```python
from build123d import *

# Parameters (mm, degrees)
BOSS_EXTRUDE1_DEPTH   = 3.81
LPATTERN1_COUNT       = 2
LPATTERN1_PITCH       = 60.96
BODY_MOVE_COPY1_ANGLE = 180
LPATTERN2_COUNT       = 3
LPATTERN2_PITCH       = 146.05
BODY_MOVE_COPY2_ANGLE = 120
BODY_MOVE_COPY3_ANGLE = 120
BOSS_EXTRUDE2_START   = -63.5
SKETCH2_R             = 9.5
BOSS_EXTRUDE2_DEPTH   = 480.06


with BuildPart() as part:
    # Sketch1 → Boss-Extrude1 (new, symmetric)
    with BuildSketch(Plane(origin=(0, 0, 0), x_dir=(1, 0, 0), z_dir=(0, 1, 0))):
        with BuildLine():
            Line((-5.499261314, 15.875), (-10.998522628, 6.35))
            ThreePointArc((-10.998522628, 6.35), (0, -12.7), (10.998522628, 6.35))
            Line((10.998522628, 6.35), (5.499261314, 15.875))
            ThreePointArc((5.499261314, 15.875), (0, 19.05), (-5.499261314, 15.875))
        make_face()
    extrude(amount=BOSS_EXTRUDE1_DEPTH, both=True)


with BuildPart() as lpattern1_1:
    # LPattern1: pattern copy
    add(part.part.moved(Location(Vector(0, 1, 0) * (1 * LPATTERN1_PITCH))))


with BuildPart() as lpattern1_1_1:
    # Body-Move/Copy1: moved
    add(lpattern1_1.part.rotate(Axis((0, 0, 0), (0, 1, 0)), BODY_MOVE_COPY1_ANGLE))


with BuildPart() as lpattern2_1:
    # LPattern2: pattern copy
    add(part.part.moved(Location(Vector(0, 1, 0) * (1 * LPATTERN2_PITCH))))


with BuildPart() as lpattern2_2:
    # LPattern2: pattern copy
    add(part.part.moved(Location(Vector(0, 1, 0) * (2 * LPATTERN2_PITCH))))


with BuildPart() as lpattern2_3:
    # LPattern2: pattern copy
    add(lpattern1_1_1.part.moved(Location(Vector(0, 1, 0) * (1 * LPATTERN2_PITCH))))


with BuildPart() as lpattern2_4:
    # LPattern2: pattern copy
    add(lpattern1_1_1.part.moved(Location(Vector(0, 1, 0) * (2 * LPATTERN2_PITCH))))


with BuildPart() as lpattern2_3_1:
    # Body-Move/Copy2: moved
    add(lpattern2_3.part.rotate(Axis((0, 0, 0), (0, 1, 0)), BODY_MOVE_COPY2_ANGLE))


with BuildPart() as lpattern2_1_1:
    # Body-Move/Copy2: moved
    add(lpattern2_1.part.rotate(Axis((0, 0, 0), (0, 1, 0)), BODY_MOVE_COPY2_ANGLE))


with BuildPart() as lpattern2_4_1:
    # Body-Move/Copy3: moved
    add(lpattern2_4.part.rotate(Axis((0, 0, 0), (0, -1, 0)), BODY_MOVE_COPY3_ANGLE))


with BuildPart() as lpattern2_2_1:
    # Body-Move/Copy3: moved
    add(lpattern2_2.part.rotate(Axis((0, 0, 0), (0, -1, 0)), BODY_MOVE_COPY3_ANGLE))


with BuildPart() as part_1:
    add(part.part)

    # Sketch2 → Boss-Extrude2 (add)
    with BuildSketch(Plane(origin=(0, 0, 0), x_dir=(1, 0, 0), z_dir=(0, 1, 0)).offset(BOSS_EXTRUDE2_START)):
        Circle(SKETCH2_R)
    extrude(amount=BOSS_EXTRUDE2_DEPTH)


with BuildPart() as lpattern1_1_2:
    add(lpattern1_1_1.part)

    # Combine1: union LPattern2_3, LPattern2_1, LPattern2_4, LPattern2_2, part
    add(lpattern2_3_1.part)
    add(lpattern2_1_1.part)
    add(lpattern2_4_1.part)
    add(lpattern2_2_1.part)
    add(part_1.part)


solid = lpattern1_1_2.part
```
Source: CAD feature listing. Evaluate the final solid. Frame: model axes, mm. A direction names the side the tool comes from. Give positions to 0.01 mm unless a question says otherwise; leave off trailing zeros. Loops run counter-clockwise (first coordinate to the right, second up) from the corner with the lowest first, then second, coordinate; pieces in that order, holes last. Notation, with made-up numbers: (70, 3.5) -> (75, 3.5) arc R24 cw to (75, 38.5) -> close; hole circle Ø6 at (-2, 35.25). An arc over 180 degrees is marked (long way). Put each result on its own line as item: value. Start each with the question number.
1) Draft query along Y for faces 5 (the face through (9, 210.82, -4)), 6 (the face through (-13.71, 146.1, -1.65)), 7 (the face through (0, 416.56, 0)). Return one class per face: released by +Y, released by -Y, zero draft, split by the parting line, or undercut.
2) Contact query for flat-ended pins moving along their axis: P1, Ø5, axis at x = 8.5, y = 312, coming from the +Z side; P2, Ø1, axis at x = 0, y = -5.5, coming from the -Z side; P3, Ø8, axis at y = 49, z = 1.5, coming from the +X side; P4, Ø5, axis at y = 189, z = -14, coming from the -X side. Output: stop coordinate, or through.
3) Reachability of faces 1 (the face through (6, 207, -12.7)), 2 (the face through (4.38, 386.3, 8.43)), 3 (the face through (8.287, 0.053, -11.046)), 4 (the face through (-1, 64.77, 10)) from +Z, -Z, +X, -X, +Y, -Y: full face, straight path, thin tool, end or side. Return the list, or none.
4) Cut plane A-A (y = 176.5). Return loops of the section in (x, z).
5) Material intervals for probe 1 along Y at (x, z) = (2.5, -11); probe 2 along Y at (x, z) = (-15, 3.5); probe 3 along Z at (x, y) = (0.5, 123.5), sorted ascending.
Results are:
1. face 5: undercut
1. face 6: zero draft
1. face 7: released by +Y
2. P1: stops at z = 7.37
2. P2: stops at z = -9.5
2. P3: stops at x = 9.5
2. P4: passes through
3. face 1: -Z, +X, -X, +Y
3. face 2: +Y
3. face 3: -Z, +X, -Y
3. face 4: none
4. outline: circle Ø19 at (0, 0)
5. probe 1: y = -3.81 to 3.81, 57.15 to 64.77, 142.24 to 149.86, 203.2 to 210.82, 288.29 to 295.91, 349.25 to 356.87
5. probe 2: y = 142.24 to 149.86
5. probe 3: z = -9.49 to 9.49
